```python
from build123d import *
from OCP.BRepFilletAPI import BRepFilletAPI_MakeChamfer

# Parameters (mm, degrees)
SKETCH2_W           = 43.4
SKETCH2_H           = 43.4
BOSS_EXTRUDE1_DEPTH = 1.56
SKETCH3_W           = 23
SKETCH3_H           = 15.6
BOSS_EXTRUDE2_DEPTH = 25
SKETCH3_3_R         = 4
SKETCH3_3_W         = 7.85
SKETCH3_3_H         = 10
SKETCH3_3_W_2       = 15
SKETCH3_3_H_2       = 7.85
SKETCH3_3_W_3       = 23
SKETCH3_3_H_3       = 15.6
BOSS_EXTRUDE3_DEPTH = 10
CHAMFER1_SIZE       = 1.3
CHAMFER1_SIZE2      = 4.85166605
SKETCH3_4_R         = 1.425
CUT_EXTRUDE1_DEPTH  = 67.273071454


with BuildPart() as part:
    # Sketch2 → Boss-Extrude1 (new body)
    with BuildSketch(Plane(origin=(0, 0, 0), x_dir=(1, 0, 0), z_dir=(0, 1, 0))):
        with Locations((21.7, 21.7)):
            Rectangle(SKETCH2_W, SKETCH2_H)
    extrude(amount=BOSS_EXTRUDE1_DEPTH)

    # Sketch3 → Boss-Extrude2 (add)
    with BuildSketch(Plane(origin=(0, 1.56, 0), x_dir=(1, 0, 0), z_dir=(0, 1, 0))):
        with Locations((21.7, 35.6)):
            Rectangle(SKETCH3_W, SKETCH3_H)
    extrude(amount=BOSS_EXTRUDE2_DEPTH)

    # Sketch3<3> → Boss-Extrude3 (add)
    with BuildSketch(Plane(origin=(0, 1.56, 0), x_dir=(1, 0, 0), z_dir=(0, 1, 0))):
        with Locations(Location((15, 17, 0), (0, 0, 90))):
            Circle(SKETCH3_3_R)
        with Locations((3.925, 15)):
            Rectangle(SKETCH3_3_W, SKETCH3_3_H)
        with Locations((13.75, 3.925)):
            Rectangle(SKETCH3_3_W_2, SKETCH3_3_H_2)
        with Locations(Location((28.9, 10.5, 0), (0, 0, 90))):
            Circle(SKETCH3_3_R)
        with Locations((39.475, 15)):
            Rectangle(SKETCH3_3_W, SKETCH3_3_H)
        with Locations((21.7, 35.6)):
            Rectangle(SKETCH3_3_W_3, SKETCH3_3_H_3)
    extrude(amount=BOSS_EXTRUDE3_DEPTH)

    # Chamfer1: one chamfer whose edges measure the first distance from different faces: ONE call of the kernel's chamfer builder (chamfer() names one face for all edges)
    chamfer1_edges_1 = [part.edges().sort_by_distance(p)[0] for p in [
        (35.55, 11.56, -15),
        (43.4, 11.56, -15),
    ]]
    chamfer1_side_1 = [part.faces().sort_by_distance(p)[0] for p in [
        (39.475, 11.56, -15),
    ]]
    chamfer1_edges_2 = [part.edges().sort_by_distance(p)[0] for p in [
        (13.75, 11.56, -7.85),
        (13.75, 11.56, 0),
    ]]
    chamfer1_side_2 = [part.faces().sort_by_distance(p)[0] for p in [
        (13.75, 11.56, -3.925),
    ]]
    chamfer1_edges_3 = [part.edges().sort_by_distance(p)[0] for p in [
        (7.85, 11.56, -15),
        (0, 11.56, -15),
    ]]
    chamfer1_side_3 = [part.faces().sort_by_distance(p)[0] for p in [
        (3.925, 11.56, -15),
    ]]
    chamfer1 = BRepFilletAPI_MakeChamfer(part.part.solid().wrapped)
    for e in chamfer1_edges_1:
        chamfer1.Add(CHAMFER1_SIZE, CHAMFER1_SIZE2, e.wrapped, chamfer1_side_1[0].wrapped)  # the first distance lies on this face
    for e in chamfer1_edges_2:
        chamfer1.Add(CHAMFER1_SIZE, CHAMFER1_SIZE2, e.wrapped, chamfer1_side_2[0].wrapped)  # the first distance lies on this face
    for e in chamfer1_edges_3:
        chamfer1.Add(CHAMFER1_SIZE, CHAMFER1_SIZE2, e.wrapped, chamfer1_side_3[0].wrapped)  # the first distance lies on this face
    add(Compound.cast(chamfer1.Shape()), mode=Mode.REPLACE)

    # Sketch3<4> → Cut-Extrude1 (cut, through all)
    with BuildSketch(Plane(origin=(0, 1.56, 0), x_dir=(1, 0, 0), z_dir=(0, 1, 0))):
        with Locations(Location((3.325, 40.075, 0), (0, 0, 270))):
            Circle(SKETCH3_4_R)
        with Locations(Location((40.075, 40.075, 0), (0, 0, 270))):
            Circle(SKETCH3_4_R)
        with Locations(Location((40.075, 3.325, 0), (0, 0, 270))):
            Circle(SKETCH3_4_R)
        with Locations(Location((3.325, 3.325, 0), (0, 0, 270))):
            Circle(SKETCH3_4_R)
    extrude(amount=-CUT_EXTRUDE1_DEPTH, mode=Mode.SUBTRACT)


solid = part.part
```
Work out the finished part from the listing and answer in its coordinate system (mm). A direction names the side the tool comes from. Give positions to 0.01 mm unless a question says otherwise; leave off trailing zeros. Order: outer loops, then holes, each group sorted by start corner. A loop starts at its lowest first (then second) coordinate and runs counter-clockwise, first axis right, second up. Notation, with made-up numbers: (46, 84.5) -> (83, 84.5) arc R36 cw to (83, 120.5) -> close; hole circle Ø7 at (60, 43.25). An arc over 180 degrees is marked (long way). Answer as CSV lines item,"result". Start each with the question number.
(1) Each of these flat-tipped pins is pushed along its axis until it touches: pin 1 Ø2.5 at (x, y) = (39, 4) entering from +Z; pin 2 Ø4 at (y, z) = (5.5, -5.5) entering from -X; pin 3 Ø4 at (y, z) = (12.5, -9) entering from +X. Where does it stop, or does it pass through?
(2) Which of the six approach directions +Z, -Z, +X, -X, +Y, -Y give full straight-line access (tool end or side, diameter ignored) to faces 1 (the flat face through (7.85, 4, -15)), 2 (the flat face through (15, 11.56, -17)), 3 (the cylindrical face through (32.805, 6.49, -9.633))?
(3) Section C-C, the plane x = 28.9 is taken. Write down the section's boundary in (y, z), plus the area to 3 significant figures.
(4) Section A-A, the plane y = 6 is taken. Write down the section's boundary in (x, z).
(5) Section B-B, the plane z = -17 is taken. Write down the section's boundary in (x, y), plus the area to 3 significant figures.
(6) Section D-D, the plane y = 19.5 is taken. Write down the section's boundary in (x, z), plus the area to 3 significant figures.
(7) For a pull along X with two mould halves and no side action, classify faces 4 (the cylindrical face through (12.3, 6.49, -14.05)), 5 (the flat face through (4, 11.56, -15)), 6 (the flat face through (0, 2, -17)) as released by +X, released by -X, zero draft, split by the parting line, or undercut.
(8) Consider line 1 along Z through (x, y) = (30, 25); line 2 along Y through (x, z) = (31, -4.5); line 3 along X through (y, z) = (19.75, -29). Determine where each line is inside the solid, lowest interval first.
Entries:
1,pin 1,"z = -10"
1,pin 2,"x = 6.25"
1,pin 3,"x = 42.31"
2,face 1,"-Z, +Y"
2,face 2,"+Z, +X, -X, +Y"
2,face 3,"+Y"
3,outline,"(0, -43.4) -> (26.56, -43.4) -> (26.56, -27.8) -> (1.56, -27.8) -> (1.56, -14.5) -> (11.56, -14.5) -> (11.56, -6.5) -> (1.56, -6.5) -> (1.56, 0) -> (0, 0) -> close"
3,area,"538 mm²"
4,outline,"(0, -20) -> (7.85, -20) -> (7.85, -10) -> (0, -10) -> close; (6.25, -7.85) -> (21.25, -7.85) -> (21.25, 0) -> (6.25, 0) -> close; (10.2, -43.4) -> (33.2, -43.4) -> (33.2, -27.8) -> (10.2, -27.8) -> close; circle Ø8 at (15, -17); circle Ø8 at (28.9, -10.5); (35.55, -20) -> (43.4, -20) -> (43.4, -10) -> (35.55, -10) -> close"
5,outline,"(0, 0) -> (43.4, 0) -> (43.4, 6.71) -> (42.1, 11.56) -> (36.85, 11.56) -> (35.55, 6.71) -> (35.55, 1.56) -> (19, 1.56) -> (19, 11.56) -> (11, 11.56) -> (11, 1.56) -> (7.85, 1.56) -> (7.85, 6.71) -> (6.55, 11.56) -> (1.3, 11.56) -> (0, 6.71) -> close"
5,area,"292 mm²"
6,outline,"(10.2, -43.4) -> (33.2, -43.4) -> (33.2, -27.8) -> (10.2, -27.8) -> close"
6,area,"359 mm²"
7,face 4,"undercut"
7,face 5,"zero draft"
7,face 6,"released by -X"
8,line 1,"-43.4 to -27.8"
8,line 2,"0 to 1.56"
8,line 3,"10.2 to 33.2"
